```python
from build123d import *

# Parameters (mm, degrees)
F0_W     = 150
F0_H     = 150
F1_DEPTH = 150
F2_R     = 15
F3_DEPTH = 150
F4_R     = 15
F5_DEPTH = 150
F6_R     = 5


with BuildPart() as f1:
    # F0 (on Front) → F1 (new body)
    with BuildSketch(Plane.XZ):
        Rectangle(F0_W, F0_H)
    extrude(amount=F1_DEPTH)

    # F2 (on face) → F3 (cut)
    with BuildSketch(Plane.XY.offset(75)):
        with Locations((0, -75)):
            Circle(F2_R)
    extrude(amount=-F3_DEPTH, mode=Mode.SUBTRACT)

    # F4 (on face) → F5 (cut)
    with BuildSketch(Plane(origin=(-75, 0, 0), x_dir=(0, -1, 0), z_dir=(-1, 0, 0))):
        with Locations((75, 0)):
            Circle(F4_R)
    extrude(amount=-F5_DEPTH, mode=Mode.SUBTRACT)

    # F6
    f6_edges = [f1.edges().sort_by_distance(p)[0] for p in [
        (75, -75, 75),
        (0, 0, 75),
        (0, -150, 75),
        (-75, -75, 75),
        (-15, -75, 75),
    ]]
    fillet(f6_edges, radius=F6_R)


solid = f1.part
```
Input: part model. Units: mm. Frame: model coordinates. Round coordinates to 2 decimals unless told otherwise and drop trailing zeros. Loops run counter-clockwise (first coordinate to the right, second up) from the corner with the lowest first, then second, coordinate; pieces in that order, holes last. Notation, with made-up numbers: (29, -2) -> (80, -2) arc R30 ccw to (80, 30) -> close; hole circle Ø10 at (55, -19). An arc over 180 degrees is marked (long way). Write each question's results on one line, items separated by ' | '.
1. Ray query, line 1 (Z direction, x = 21, y = -75); line 2 (Y direction, x = 0, z = 31). Return the intervals inside material, ascending. Write a range as from..to.
Geometry results:
line 1: -75..-15, 15..75 | line 2: -150..-90, -60..0
2. Section B-B (x = 61.5). Return loops of the section in (y, z).
Geometry results:
outline: (-150, -75) -> (0, -75) -> (0, 70) arc R5 ccw to (-5, 75) -> (-145, 75) arc R5 ccw to (-150, 70) -> close; hole circle Ø30 at (-75, 0)
3. Mould query, pull axis Y, two halves, no side actions, for faces 1 (the face through (-1, -150, -1)), 2 (the face through (73, -76, 74)), 3 (the face through (-1, 0, -1)), 4 (the face through (-46.358, -73.047, 14.872)). Classes: +Y half, -Y half, draft (parallel to the pull), parting line (faces both ways), or undercut.
Geometry results:
face 1: -Y half | face 2: draft | face 3: +Y half | face 4: undercut
4. Section C-C (z = -19.5). Return loops of the section in (x, y).
Geometry results:
outline: (-75, -150) -> (75, -150) -> (75, 0) -> (-75, 0) -> close; hole circle Ø30 at (0, -75)
5. Section A-A (y = -75). Return loops of the section in (x, z).
Geometry results:
outline: (-75, -75) -> (-15, -75) -> (-15, -15) -> (-75, -15) -> close; (-75, 15) -> (-15, 15) -> (-15, 70) arc R5 ccw to (-20, 75) -> (-70, 75) arc R5 ccw to (-75, 70) -> close; (15, -75) -> (75, -75) -> (75, -15) -> (15, -15) -> close; (15, 15) -> (75, 15) -> (75, 70) arc R5 ccw to (70, 75) -> (20, 75) arc R5 ccw to (15, 70) -> close
6. First-contact query: P1, Ø18, axis at x = 0, y = -75, coming from the -Z side. Flat tip, straight axial feed; report the tip coordinate or a pass-through.
Geometry results:
P1: through
